```python
from build123d import *

# Parameters (mm, degrees)
SALIENTE_EXTRUIR1_DEPTH = 1.95
CROQUIS2_W              = 9.2
CROQUIS2_H              = 12
CORTAR_EXTRUIR1_DEPTH   = 2


with BuildPart() as part:
    # Croquis1 → Saliente-Extruir1 (new body)
    with BuildSketch(Plane.XY):
        with BuildLine():
            Line((0, 0), (-12, 0))
            Line((-12, 0), (-12, 9.5341439))
            ThreePointArc((-12, 9.5341439), (-15.903544777, 12.873087069), (-18.1346611, 17.5))
            Line((-18.1346611, 17.5), (-26.5, 17.5))
            Line((-26.5, 17.5), (-26.5, 23.5))
            Line((-26.5, 23.5), (-18.1346611, 23.5))
            ThreePointArc((-18.1346611, 23.5), (-14.838834765, 29.338834765), (-9, 32.6346611))
            Line((-9, 32.6346611), (-9, 41))
            Line((-9, 41), (-3, 41))
            Line((-3, 41), (-3, 32.6346611))
            ThreePointArc((-3, 32.6346611), (2.838834765, 29.338834765), (6.1346611, 23.5))
            Line((6.1346611, 23.5), (14.5, 23.5))
            Line((14.5, 23.5), (14.5, 17.5))
            Line((14.5, 17.5), (6.1346611, 17.5))
            ThreePointArc((6.1346611, 17.5), (3.903544777, 12.873087069), (0, 9.5341439))
            Line((0, 9.5341439), (0, 0))
        make_face()
        with BuildLine():
            Line((-9, 23.5), (-9, 27.373863542))
            ThreePointArc((-9, 27.373863542), (-11.303300859, 25.803300859), (-12.873863542, 23.5))
            Line((-12.873863542, 23.5), (-9, 23.5))
        make_face(mode=Mode.SUBTRACT)
        with BuildLine():
            Line((-3, 23.5), (-3, 27.373863542))
            ThreePointArc((-3, 27.373863542), (-0.696699141, 25.803300859), (0.873863542, 23.5))
            Line((0.873863542, 23.5), (-3, 23.5))
        make_face(mode=Mode.SUBTRACT)
        with BuildLine():
            Line((-9, 17.5), (-9, 13.626136458))
            ThreePointArc((-9, 13.626136458), (-11.303300859, 15.196699141), (-12.873863542, 17.5))
            Line((-12.873863542, 17.5), (-9, 17.5))
        make_face(mode=Mode.SUBTRACT)
        with BuildLine():
            Line((-3, 17.5), (-3, 13.626136458))
            ThreePointArc((-3, 13.626136458), (-0.696699141, 15.196699141), (0.873863542, 17.5))
            Line((0.873863542, 17.5), (-3, 17.5))
        make_face(mode=Mode.SUBTRACT)
    extrude(amount=SALIENTE_EXTRUIR1_DEPTH)

    # Croquis2 → Cortar-Extruir1 (cut)
    with BuildSketch(Plane.XY.offset(4)):
        with Locations((-6, 6)):
            Rectangle(CROQUIS2_W, CROQUIS2_H)
    extrude(amount=-CORTAR_EXTRUIR1_DEPTH, mode=Mode.SUBTRACT)


solid = part.part
```
Work out the finished part from the listing and answer in its coordinate system (mm). A direction names the side the tool comes from. Give positions to 0.01 mm unless a question says otherwise; leave off trailing zeros. Loops run counter-clockwise (first coordinate to the right, second up) from the corner with the lowest first, then second, coordinate; pieces in that order, holes last. Notation, with made-up numbers: M 64.5,-20.75 L 92.5,-20.75 A15 cw 92.5,5.25 Z; hole C -25,51.25 d5. An arc over 180 degrees is marked long. One line per item, written item: value. Start each with the question number.
1. Find section C-C (y = 35). Give the vertices of the cut face in (x, z).
2. Determine the mould class of faces 1 (the face through (-9, 25, 1)), 2 (the face through (0, 5, 1)), 3 (the face through (-0.725, 15.169, 0.961)), 4 (the face through (-6, 41, 1)) for opening direction X: released by +X, released by -X, zero draft, split by the parting line, or undercut.
3. Find section A-A (z = 0.5). Give the vertices of the cut face in (x, y).
4. Which of the six approach directions +Z, -Z, +X, -X, +Y, -Y give full straight-line access (tool end or side, diameter ignored) to faces 5 (the face through (10, 17.5, 1)), 6 (the face through (-1, 17.5, 1)), 7 (the face through (-9, 37, 1))?
5. Find section B-B (y = 16.5). Give the vertices of the cut face in (x, z).
6. Find section D-D (x = 4). Give the vertices of the cut face in (y, z).
7. Find the intervals of material crossed by probe 1 along Y at (x, z) = (-10, 1.05); probe 2 along X at (y, z) = (27, 0.4); probe 3 along Y at (x, z) = (12.5, 1), in increasing order.
8. Each of these flat-tipped pins is pushed along its axis until it touches: P1, Ø0.6, axis at y = 26, z = 0.5, coming from the +X side; P2, Ø0.6, axis at x = 10.5, z = 0.5, coming from the +Y side; P3, Ø0.6, axis at x = -10.5, z = 1, coming from the +Y side. Where does it stop, or does it pass through?
Reported:
1. outline: M -9,0 L -3,0 L -3,1.95 L -9,1.95 Z
2. face 1: undercut
2. face 2: released by +X
2. face 3: undercut
2. face 4: zero draft
3. outline: M -26.5,17.5 L -18.13,17.5 A12.5 ccw -12,9.53 L -12,0 L 0,0 L 0,9.53 A12.5 ccw 6.13,17.5 L 14.5,17.5 L 14.5,23.5 L 6.13,23.5 A12.5 ccw -3,32.63 L -3,41 L -9,41 L -9,32.63 A12.5 ccw -18.13,23.5 L -26.5,23.5 Z; hole M -12.87,17.5 A7.5 ccw -9,13.63 L -9,17.5 Z; hole M -12.87,23.5 L -9,23.5 L -9,27.37 A7.5 ccw Z; hole M -3,13.63 A7.5 ccw 0.87,17.5 L -3,17.5 Z; hole M -3,23.5 L 0.87,23.5 A7.5 ccw -3,27.37 Z
4. face 5: +Z, -Z, +X, -Y
4. face 6: +Z, -Z
4. face 7: +Z, -Z, -X, +Y
5. outline: M -17.84,0 L -12.34,0 L -12.34,1.95 L -17.84,1.95 Z; M -9,0 L -3,0 L -3,1.95 L -9,1.95 Z; M 0.34,0 L 5.84,0 L 5.84,1.95 L 0.34,1.95 Z
6. outline: M 13,0 L 28,0 L 28,1.95 L 13,1.95 Z
7. probe 1: y = 0 to 14.16, 17.5 to 23.5, 26.84 to 32.34
7. probe 2: x = -16.68 to -9.74, -9 to -3, -2.26 to 4.68
7. probe 3: y = 17.5 to 23.5
8. P1: stops at x = 5.37
8. P2: stops at y = 23.5
8. P3: stops at y = 32.27
